```python
from build123d import *

# Parameters (mm, degrees)
SKETCH1_R           = 1.15
BOSS_EXTRUDE1_DEPTH = 1.4
BOSS_EXTRUDE2_START = -1.4
SKETCH2_R           = 3.95
BOSS_EXTRUDE2_DEPTH = 9
SKETCH3_W           = 4.2
SKETCH3_H           = 11.7
BOSS_EXTRUDE4_DEPTH = 8.6
SKETCH4_W           = 3.3
SKETCH4_H           = 9
CUT_EXTRUDE1_DEPTH  = 7
SKETCH5_W           = 0.45
SKETCH5_H           = 6.4
CUT_EXTRUDE2_DEPTH  = 2.8
SKETCH6_W           = 3.777009852
SKETCH6_H           = 2.7350761
BOSS_EXTRUDE6_DEPTH = 3.3
SKETCH7_W           = 4.5
SKETCH7_H           = 4.5
BOSS_EXTRUDE7_DEPTH = 1.1
SKETCH8_R           = 2.35
CUT_EXTRUDE3_DEPTH  = 0.1


with BuildPart() as part:
    # Sketch1 → Boss-Extrude1 (new body)
    with BuildSketch(Plane(origin=(0, 0, 0), x_dir=(1, 0, 0), z_dir=(0, 1, 0))):
        with BuildLine():
            Line((25.738550612, -3.990919322), (25.738550612, -12.04368231))
            Line((25.738550612, -12.04368231), (18.338550612, -12.04368231))
            ThreePointArc((18.338550612, -12.04368231), (15.838550612, -9.54368231), (13.338550612, -12.04368231))
            Line((13.338550612, -12.04368231), (-3.061449388, -12.04368231))
            ThreePointArc((-3.061449388, -12.04368231), (-5.011449388, -13.99368231), (-6.961449388, -12.04368231))
            Line((-6.961449388, -12.04368231), (-14.561449388, -12.04368231))
            Line((-14.561449388, -12.04368231), (-14.561449388, -4.543434765))
            ThreePointArc((-14.561449388, -4.543434765), (-12.096629884, -2.04368231), (-14.561449388, 0.456070144))
            Line((-14.561449388, 0.456070144), (-14.561449388, 7.85631769))
            Line((-14.561449388, 7.85631769), (-6.961449388, 7.85631769))
            ThreePointArc((-6.961449388, 7.85631769), (-5.011449388, 9.80631769), (-3.061449388, 7.85631769))
            Line((-3.061449388, 7.85631769), (13.338550612, 7.85631769))
            ThreePointArc((13.338550612, 7.85631769), (15.838550612, 5.35631769), (18.338550612, 7.85631769))
            Line((18.338550612, 7.85631769), (25.738550612, 7.85631769))
            Line((25.738550612, 7.85631769), (25.738550612, -0.096445299))
            ThreePointArc((25.738550612, -0.096445299), (27.792319693, -2.04368231), (25.738550612, -3.990919322))
        make_face()
        with Locations((25.842319693, -2.04368231)):
            Circle(SKETCH1_R, mode=Mode.SUBTRACT)
        with Locations((-5.011449388, -12.04368231)):
            Circle(SKETCH1_R, mode=Mode.SUBTRACT)
        with Locations((-5.011449388, 7.85631769)):
            Circle(SKETCH1_R, mode=Mode.SUBTRACT)
    extrude(amount=BOSS_EXTRUDE1_DEPTH)

    # Sketch2 → Boss-Extrude2 (add)
    with BuildSketch(Plane(origin=(0, 1.4, 0), x_dir=(1, 0, 0), z_dir=(0, 1, 0)).offset(BOSS_EXTRUDE2_START)):
        with Locations((19.742319693, -2.04368231)):
            Circle(SKETCH2_R)
    extrude(amount=BOSS_EXTRUDE2_DEPTH)

    # Sketch3 → Boss-Extrude4 (add)
    with BuildSketch(Plane(origin=(0, 1.4, 0), x_dir=(1, 0, 0), z_dir=(0, 1, 0))):
        with Locations((-10.761449388, -2.04368231)):
            Rectangle(SKETCH3_W, SKETCH3_H)
    extrude(amount=BOSS_EXTRUDE4_DEPTH)

    # Sketch4 → Cut-Extrude1 (cut)
    with BuildSketch(Plane(origin=(0, 10, 0), x_dir=(1, 0, 0), z_dir=(0, 1, 0))):
        with Locations((-10.761449388, -2.04368231)):
            Rectangle(SKETCH4_W, SKETCH4_H)
    extrude(amount=-CUT_EXTRUDE1_DEPTH, mode=Mode.SUBTRACT)

    # Sketch5 → Cut-Extrude2 (cut)
    with BuildSketch(Plane(origin=(0, 10, 0), x_dir=(1, 0, 0), z_dir=(0, 1, 0))):
        with Locations((-8.886449388, -2.04368231)):
            Rectangle(SKETCH5_W, SKETCH5_H)
    extrude(amount=-CUT_EXTRUDE2_DEPTH, mode=Mode.SUBTRACT)

    # Sketch6 → Boss-Extrude6 (add)
    with BuildSketch(Plane(origin=(0, 1.4, 0), x_dir=(1, 0, 0), z_dir=(0, 1, 0))):
        Polygon((-7.884809568, 6.198373802), (-2.023932211, 6.198373802), (-2.023932211, 4.895956612), (17.251842208, 4.895956612), (17.251842208, 1.987224886), (14.169454857, 1.987224886), (14.169454857, -8.866251701), (12.085587353, -8.866251701), (12.085587353, -11.210602644), (0.320418732, -11.210602644), (0.320418732, -6.000933882), (-7.884809568, -6.000933882), align=None)
        with Locations((23.134426518, 5.482044347)):
            Rectangle(SKETCH6_W, SKETCH6_H)
    extrude(amount=BOSS_EXTRUDE6_DEPTH)

    # Sketch7 → Boss-Extrude7 (add)
    with BuildSketch(Plane.XZ):
        with Locations((20.088550612, 2.04368231)):
            Rectangle(SKETCH7_W, SKETCH7_H)
    extrude(amount=BOSS_EXTRUDE7_DEPTH)

    # Sketch8 → Cut-Extrude3 (cut)
    with BuildSketch(Plane(origin=(0, 9, 0), x_dir=(1, 0, 0), z_dir=(0, 1, 0))):
        with Locations((19.742319693, -2.04368231)):
            Circle(SKETCH8_R)
    extrude(amount=-CUT_EXTRUDE3_DEPTH, mode=Mode.SUBTRACT)


solid = part.part
```
Here's how the part is built. I have some questions about the finished solid (model axes, mm). A direction names the side the tool comes from. Round coordinates to 2 decimals unless told otherwise and drop trailing zeros. Write each loop counter-clockwise with the first axis right and the second up, starting at its lowest first coordinate (ties: lowest second). Pieces come first, ordered by that corner, then holes.
Q1. Please list where these lines run through material, in increasing order: probe 1 along X at (y, z) = (7, 1); probe 2 along Z at (x, y) = (-4.5, 0.5); probe 3 along X at (y, z) = (4.5, 4.25).
Q2. If we section it at C-C on x = 20.5: Write out the boundary of the cut face in (y, z), plus the area to 3 significant figures.
Q3. Will these pins go through, and if not, where does the flat tip stop? P1, Ø4, axis at x = -2, z = 4.5, coming from the -Y side; P2, Ø1.5, axis at y = 7.5, z = 4.5, coming from the +X side; P3, Ø1, axis at y = 3, z = 8.5, coming from the -X side.
Q4. If we section it at A-A on y = 6.75: Write out the boundary of the cut face in (x, z).
Q5. If we section it at B-B on z = -3.25: Write out the boundary of the cut face in (x, y).
Q6. If we mould it in two halves opening along X, with no side actions, what happens to faces 5 (the flat face through (22, 1, -7.856)), 6 (the flat face through (17.839, -0.5, 2)), 7 (the flat face through (-8.661, 5, 2)), 8 (the flat face through (25.739, 1, 8))? For each: +X half, -X half, draft (parallel to the pull), parting line (faces both ways), or undercut.
Q7. Which directions (+Z, -Z, +X, -X, +Y, -Y) give clear straight access to the entire face, cutting with the end or side of a thin tool? Please do faces 1 (the flat face through (14.169, 3, 3)), 2 (the flat face through (20.1, -0.5, -0.206)), 3 (the flat face through (23, 3, -6.85)), 4 (the cylindrical face through (15.796, 5.147, 1.87)).
Answer below:
1. probe 1: x = -12.86 to -12.41, -9.11 to -8.66, 15.93 to 23.55
1. probe 2: z = -9.74 to -8.89, -6.83 to 11.01, 13.07 to 13.93
1. probe 3: x = -12.86 to -12.41, -9.11 to -8.66, -7.88 to 14.17, 16.47 to 23.02
2. outline: (-1.1, -0.21) - (0, -0.21) - (0, -7.86) - (1.4, -7.86) - (1.4, -1.83) - (9, -1.83) - (9, -0.18) - (8.9, -0.18) - (8.9, 4.27) - (9, 4.27) - (9, 5.92) - (1.4, 5.92) - (1.4, 12.04) - (0, 12.04) - (0, 4.29) - (-1.1, 4.29) - close
2. area: 91.3 mm2
3. P1: stops at y = 0
3. P2: stops at x = 23.3
3. P3: stops at x = 0.32
4. outline: (-12.86, -3.81) - (-8.66, -3.81) - (-8.66, 7.89) - (-12.86, 7.89) - close; circle Ø7.9 at (19.74, 2.04); hole (-12.41, -2.46) - (-9.11, -2.46) - (-9.11, 6.54) - (-12.41, 6.54) - close
5. outline: (-14.56, 0) - (25.74, 0) - (25.74, 1.4) - (17.25, 1.4) - (17.25, 4.7) - (-7.88, 4.7) - (-7.88, 1.4) - (-8.66, 1.4) - (-8.66, 10) - (-12.86, 10) - (-12.86, 1.4) - (-14.56, 1.4) - close
6. face 5: draft
6. face 6: -X half
6. face 7: undercut
6. face 8: +X half
7. face 1: +Z, +Y
7. face 2: -Z, +X, -X, -Y
7. face 3: -Z, +X, -X, +Y
7. face 4: +Y
